The model under review builds one solid part; all positions refer to its coordinate system, in mm. A direction names the side the tool comes from. Round coordinates to 2 decimals unless told otherwise and drop trailing zeros. Order: outer loops, then holes, each group sorted by start corner. A loop starts at its lowest first (then second) coordinate and runs counter-clockwise, first axis right, second up.
1) Consider section B-B (y = -68.5). Give the boundary of the cut face in (x, z).
2) Mouldability with a two-part tool opening along Y and no side actions: class faces 1 (the face through (-125, 0.5, 27.4)), 2 (the face through (-106.171, 111.135, 1.409)), 3 (the face through (-127, 2, 23)) as pulls with the +Y half, pulls with the -Y half, needs draft (parallel to the pull), parting line crosses it, or undercut.
3) To check wall thickness, follow L1, parallel to Y at x = -126.7, z = 24; L2, parallel to X at y = -67, z = 18; L3, parallel to Z at x = 126.7, y = 0. State the ranges of each line that lie inside material, in increasing order.
4) Clearance check with flat-ended pins moving along their axes: P1, Ø2.5, axis at y = -94.29, z = 24, coming from the -X side; P2, Ø0.5, axis at x = 117, y = 110.5, coming from the +Z side; P3, Ø2.5, axis at y = 11, z = 23.5, coming from the +X side; P4, Ø8, axis at x = 91, y = 31.5, coming from the +Z side. State where each tip first meets the part, or that it passes through.
5) Consider section A-A (x = 45.5). Give the boundary of the cut face in (y, z).
6) Consider section C-C (y = 46). Give the boundary of the cut face in (x, z), then the cut area to 3 significant figures.
7) Machinability: for faces 4 (the face through (-2, 4, 0)), 5 (the face through (-127.36, 108.23, 32.19)), 6 (the face through (127, 2, 23)), which of the approach directions +Z, -Z, +X, -X, +Y, -Y give a long, thin tool a straight path to every point of the face, cutting with its end or side? Answer none if there is none.
from build123d import *

# Parameters (mm, degrees)
SKETCH1_W                                      = 255
SKETCH1_H                                      = 223
BOSS_EXTRUDE1_DEPTH                            = 2.5
SKETCH2_W                                      = 2.5
SKETCH2_H                                      = 223
SKETCH2_W_2                                    = 250
SKETCH2_H_2                                    = 2.5
BOSS_EXTRUDE2_DEPTH                            = 54
FRONT_TAPER_DEPTH                              = 178.776545135
FRONT_TAPER_DEPTH_BACK                         = 178.776545135
HOLD_IN_TAB_DEPTH                              = 3
SKETCH6_W                                      = 8.4
SKETCH6_H                                      = 227.2
MOUNTING_POCKET_DEPTH                          = 284.052115343
CSK_FOR_M3_FLAT_HEAD_MACHINE_SCREW1_AT_2_COUNT = 2
CSK_FOR_M3_FLAT_HEAD_MACHINE_SCREW1_AT_2_PITCH = 94.285714286
CSK_FOR_M3_FLAT_HEAD_MACHINE_SCREW1_AT_3_COUNT = 2
CSK_FOR_M3_FLAT_HEAD_MACHINE_SCREW1_AT_3_PITCH = 188.571428571
FILLET2_R                                      = 5
FILLET3_R                                      = 10
FILLET4_R                                      = 50
INSERT_CHAMS_SIZE                              = 1.5
INSIDE_CHAMS_SIZE                              = 2
DEBURS_SIZE                                    = 0.5


with BuildPart() as part:
    # Sketch1 → Boss-Extrude1 (new body)
    with BuildSketch(Plane.XY):
        Rectangle(SKETCH1_W, SKETCH1_H)
    extrude(amount=-BOSS_EXTRUDE1_DEPTH)

    # Sketch2 → Boss-Extrude2 (add)
    with BuildSketch(Plane.XY):
        with Locations((-126.25, 0)):
            Rectangle(SKETCH2_W, SKETCH2_H)
        with Locations((0, -110.25)):
            Rectangle(SKETCH2_W_2, SKETCH2_H_2)
        with Locations((126.25, 0)):
            Rectangle(SKETCH2_W, SKETCH2_H)
    extrude(amount=BOSS_EXTRUDE2_DEPTH)

    # Sketch5 → Front Taper (cut, two sides: drawn at the far end of the back side and taken through both)
    with BuildSketch(Plane(origin=(0, 0, 0), x_dir=(0, 0, -1), z_dir=(1, 0, 0)).offset(-FRONT_TAPER_DEPTH_BACK)):
        Polygon((-54, 31.5), (-33, 111.5), (-54, 111.5), align=None)
    extrude(amount=FRONT_TAPER_DEPTH + FRONT_TAPER_DEPTH_BACK, mode=Mode.SUBTRACT)

    # Sketch10 → Hold In Tab (add)
    with BuildSketch(Plane(origin=(0, 111.5, 0), x_dir=(1, 0, 0), z_dir=(0, 1, 0))):
        Polygon((127.5, -15), (113.5, -15), (107.5, -9), (107.5, 2.5), (127.5, 2.5), align=None)
    hold_in_tab = extrude(amount=-HOLD_IN_TAB_DEPTH)

    # Hold Tabs: Hold In Tab across plane
    add(hold_in_tab.mirror(Plane(origin=(0, 0, 0), x_dir=(0, 0, 1), z_dir=(1, 0, 0))))

    # Sketch6 → Mounting Pocket (cut, through all)
    with BuildSketch(Plane.ZY.offset(-127)):
        with Locations((24, 1.35)):
            Rectangle(SKETCH6_W, SKETCH6_H)
    mounting_pocket = extrude(amount=-MOUNTING_POCKET_DEPTH, mode=Mode.SUBTRACT)

    # Mounting Pockets: Mounting Pocket across plane
    add(mounting_pocket.mirror(Plane(origin=(0, 0, 0), x_dir=(0, 0, 1), z_dir=(1, 0, 0))), mode=Mode.SUBTRACT)

    # Sketch9 → CSK for M3 Flat Head Machine Screw1 (revolve, cut)
    with BuildSketch(Plane(origin=(125, -94.285714286, 24), x_dir=(0, 0, 1), z_dir=(0, 1, 0))):
        Polygon((0, 0), (0, 2), (1.8, 2), (1.7, 1.9), (1.7, 1.55), (3.25, 0), align=None)
    csk_for_m3_flat_head_machine_screw1 = revolve(axis=Axis((118.65, -94.285714286, 24), (1, 0, 0)), mode=Mode.SUBTRACT)

    # CSK for M3 Flat Head Machine Screw1 at 2: CSK for M3 Flat Head Machine Screw1 ×2
    with Locations(*[(0, i * CSK_FOR_M3_FLAT_HEAD_MACHINE_SCREW1_AT_2_PITCH, 0) for i in range(1, CSK_FOR_M3_FLAT_HEAD_MACHINE_SCREW1_AT_2_COUNT)]):
        add(csk_for_m3_flat_head_machine_screw1, mode=Mode.SUBTRACT)

    # CSK for M3 Flat Head Machine Screw1 at 3: CSK for M3 Flat Head Machine Screw1 ×2
    with Locations(*[(0, i * CSK_FOR_M3_FLAT_HEAD_MACHINE_SCREW1_AT_3_PITCH, 0) for i in range(1, CSK_FOR_M3_FLAT_HEAD_MACHINE_SCREW1_AT_3_COUNT)]):
        add(csk_for_m3_flat_head_machine_screw1, mode=Mode.SUBTRACT)

    # Mounting Screw Holes: CSK for M3 Flat Head Machine Screw1 across plane
    add(csk_for_m3_flat_head_machine_screw1.mirror(Plane(origin=(0, 0, 0), x_dir=(0, 0, 1), z_dir=(1, 0, 0))), mode=Mode.SUBTRACT)

    # Mounting Screw Holes copy 1 sketch → Mounting Screw Holes copy 1 (revolve, cut)
    with BuildSketch(Plane(origin=(-125, 0, 24), x_dir=(0, 0, 1), z_dir=(0, 1, 0))):
        Polygon((0, 0), (0, -2), (1.8, -2), (1.7, -1.9), (1.7, -1.55), (3.25, 0), align=None)
    revolve(axis=Axis((-118.65, 0, 24), (1, 0, 0)), mode=Mode.SUBTRACT)

    # Mounting Screw Holes copy 2 sketch → Mounting Screw Holes copy 2 (revolve, cut)
    with BuildSketch(Plane(origin=(-125, 94.285714286, 24), x_dir=(0, 0, 1), z_dir=(0, 1, 0))):
        Polygon((0, 0), (0, -2), (1.8, -2), (1.7, -1.9), (1.7, -1.55), (3.25, 0), align=None)
    revolve(axis=Axis((-118.65, 94.285714286, 24), (1, 0, 0)), mode=Mode.SUBTRACT)

    # Fillet2
    fillet2_edges = [part.edges().sort_by_distance(p)[0] for p in [
        (125, 110, 15),
        (107.5, 110, 0),
        (107.5, 110, 9),
        (113.5, 110, 15),
        (-125, 110, 15),
        (-107.5, 110, 0),
        (-107.5, 110, 9),
        (-113.5, 110, 15),
    ]]
    fillet(fillet2_edges, radius=FILLET2_R)

    # Fillet3
    fillet3_edges = [part.edges().sort_by_distance(p)[0] for p in [
        (-126.25, 111.5, 33),
        (126.25, 111.5, 33),
    ]]
    fillet(fillet3_edges, radius=FILLET3_R)

    # Fillet4
    fillet4_edges = [part.edges().sort_by_distance(p)[0] for p in [
        (126.25, 31.5, 54),
        (-126.25, 31.5, 54),
    ]]
    fillet(fillet4_edges, radius=FILLET4_R)

    # Insert Chams
    # the kernel refuses this chamfer: 1.5 mm, written as the material it takes off along each edge
    with BuildSketch(Plane(origin=(-112.035533906, 108.5, 13.535533906), x_dir=(0.01944252080601449, 0.9996219169112968, 0.01944252080601441), z_dir=(0.7071067811865461, 0, -0.707106781186549)), Plane(origin=(112.035533906, 108.5, 13.535533906), x_dir=(0.706839436070675, -0.02749587661058209, -0.7068394360706722), z_dir=(-0.7071067811865461, 0, -0.707106781186549))) as insert_chams_piece_1:
        Polygon((INSERT_CHAMS_SIZE * 0.999621916911, -INSERT_CHAMS_SIZE * 0.0274958766106), (-INSERT_CHAMS_SIZE * 0.0274958766106, -INSERT_CHAMS_SIZE * 0.999621916911), (0, 0), align=None)
    extrude(amount=4.343145751, mode=Mode.SUBTRACT)
    with BuildSketch(Plane(origin=(-107.5, 108.5, 6.928932188), x_dir=(0.027495876610582292, 0.9996219169112969, 0), z_dir=(0, 0, -1)), Plane(origin=(107.5, 108.5, 6.928932188), x_dir=(0.9996219169112969, -0.027495876610582292, 0), z_dir=(0, 0, -1))) as insert_chams_piece_2:
        Polygon((INSERT_CHAMS_SIZE * 0.999621916911, -INSERT_CHAMS_SIZE * 0.0274958766106), (-INSERT_CHAMS_SIZE * 0.0274958766106, -INSERT_CHAMS_SIZE * 0.999621916911), (0, 0), align=None)
    extrude(amount=1.928932188, mode=Mode.SUBTRACT)
    with BuildSketch(Plane(origin=(-120, 108.5, 15), x_dir=(0, 0.9996219169112968, 0.027495876610586893), z_dir=(1, 0, 0)), Plane(origin=(120, 108.5, 15), x_dir=(0, -0.027495876610582164, -0.9996219169112969), z_dir=(-1, 0, 0))) as insert_chams_piece_3:
        Polygon((INSERT_CHAMS_SIZE * 0.999621916911, -INSERT_CHAMS_SIZE * 0.0274958766106), (-INSERT_CHAMS_SIZE * 0.0274958766106, -INSERT_CHAMS_SIZE * 0.999621916911), (0, 0), align=None)
    extrude(amount=4.428932188, mode=Mode.SUBTRACT)
    with BuildSketch(Plane(origin=(-115.571067812, 108.5, 10), x_dir=(0, 0, 1), z_dir=(-1, 0, 0))) as insert_chams_piece_4:
        Polygon((5, INSERT_CHAMS_SIZE), (5 - INSERT_CHAMS_SIZE, 0), (5, 0), align=None)
    revolve(axis=Axis((-115.571067812, 108.5, 10), (0, 1, 0)), revolution_arc=45, mode=Mode.SUBTRACT)
    with BuildSketch(Plane(origin=(-112.5, 108.5, 6.928932188), x_dir=(1, 0, 0), z_dir=(0, 0, -1))) as insert_chams_piece_5:
        Polygon((5, -INSERT_CHAMS_SIZE), (5 - INSERT_CHAMS_SIZE, 0), (5, 0), align=None)
    revolve(axis=Axis((-112.5, 108.5, 6.928932188), (0, -1, 0)), revolution_arc=45, mode=Mode.SUBTRACT)
    with BuildSketch(Plane(origin=(115.571067812, 108.5, 10), x_dir=(0, 0, 1), z_dir=(1, 0, 0))) as insert_chams_piece_6:
        Polygon((5 - INSERT_CHAMS_SIZE, 0), (5, -INSERT_CHAMS_SIZE), (5, 0), align=None)
    revolve(axis=Axis((115.571067812, 108.5, 10), (0, -1, 0)), revolution_arc=45, mode=Mode.SUBTRACT)
    with BuildSketch(Plane(origin=(112.5, 108.5, 6.928932188), x_dir=(-0.7071067811865478, 0, 0.7071067811865472), z_dir=(0.7071067811865472, 0, 0.7071067811865478))) as insert_chams_piece_7:
        Polygon((5 - INSERT_CHAMS_SIZE, 0), (5, -INSERT_CHAMS_SIZE), (5, 0), align=None)
    revolve(axis=Axis((112.5, 108.5, 6.928932188), (0, -1, 0)), revolution_arc=45, mode=Mode.SUBTRACT)
    with BuildSketch(Plane(origin=(-120, 108.5, 20), x_dir=(-0.7166461305573681, 0, 0.6974369674437623), z_dir=(0.6974369674437623, 0, 0.7166461305573681))) as insert_chams_piece_8_section:
        Polygon((5, -INSERT_CHAMS_SIZE), (5 + INSERT_CHAMS_SIZE, 0), (5, 0), align=None)
    insert_chams_piece_8 = revolve(axis=Axis((-120, 108.5, 20), (0, -1, 0)), revolution_arc=134.221731534, mode=Mode.PRIVATE)
    insert_chams_piece_8 = split(insert_chams_piece_8, bisect_by=Plane(origin=(-125, 109.058393583, 16.326998509), z_dir=(1, 0, 0)), keep=Keep.TOP, mode=Mode.PRIVATE)
    add(insert_chams_piece_8, mode=Mode.SUBTRACT)
    with BuildSketch(Plane(origin=(-102.5, 108.5, 5), x_dir=(0.6974369674437586, 0, -0.7166461305573718), z_dir=(0.7166461305573718, 0, 0.6974369674437586))) as insert_chams_piece_9_section:
        Polygon((5, INSERT_CHAMS_SIZE), (5 + INSERT_CHAMS_SIZE, 0), (5, 0), align=None)
    insert_chams_piece_9 = revolve(axis=Axis((-102.5, 108.5, 5), (0, 1, 0)), revolution_arc=134.221731534, mode=Mode.PRIVATE)
    insert_chams_piece_9 = split(insert_chams_piece_9, bisect_by=Plane(origin=(-106.173001491, 109.058393583, 0), z_dir=(0, 0, 1)), keep=Keep.TOP, mode=Mode.PRIVATE)
    add(insert_chams_piece_9, mode=Mode.SUBTRACT)
    with BuildSketch(Plane(origin=(102.5, 108.5, 5), x_dir=(-0.6974369674437586, 0, -0.7166461305573718), z_dir=(-0.7166461305573718, 0, 0.6974369674437586))) as insert_chams_piece_10_section:
        Polygon((5 + INSERT_CHAMS_SIZE, 0), (5, -INSERT_CHAMS_SIZE), (5, 0), align=None)
    insert_chams_piece_10 = revolve(axis=Axis((102.5, 108.5, 5), (0, -1, 0)), revolution_arc=134.221731534, mode=Mode.PRIVATE)
    insert_chams_piece_10 = split(insert_chams_piece_10, bisect_by=Plane(origin=(106.173001491, 109.058393583, 0), z_dir=(0, 0, 1)), keep=Keep.TOP, mode=Mode.PRIVATE)
    add(insert_chams_piece_10, mode=Mode.SUBTRACT)
    with BuildSketch(Plane(origin=(120, 108.5, 20), x_dir=(0.716646130557371, 0, 0.6974369674437595), z_dir=(-0.6974369674437595, 0, 0.716646130557371))) as insert_chams_piece_11_section:
        Polygon((5, INSERT_CHAMS_SIZE), (5 + INSERT_CHAMS_SIZE, 0), (5, 0), align=None)
    insert_chams_piece_11 = revolve(axis=Axis((120, 108.5, 20), (0, 1, 0)), revolution_arc=134.221731534, mode=Mode.PRIVATE)
    insert_chams_piece_11 = split(insert_chams_piece_11, bisect_by=Plane(origin=(125, 109.058393583, 16.326998509), z_dir=(-1, 0, 0)), keep=Keep.TOP, mode=Mode.PRIVATE)
    add(insert_chams_piece_11, mode=Mode.SUBTRACT)

    # Inside Chams
    inside_chams_edges = [part.edges().sort_by_distance(p)[0] for p in [
        (-125, -109, 27),
        (125, -109, 27),
        (0, -109, 0),
        (-125, 108.5, 7.923344034),
        (-115.826655966, 108.5, 0),
        (125, 108.5, 7.923344034),
        (125, -0.25, 0),
        (115.826655966, 108.5, 0),
        (-125, -0.25, 0),
    ]]
    chamfer(inside_chams_edges, length=INSIDE_CHAMS_SIZE)

    # Deburs
    deburs_edges = [part.edges().sort_by_distance(p)[0] for p in [
        (-127.5, 0, -2.5),
        (0, -111.5, -2.5),
        (0, -111.5, 54),
        (-110.5, 111.5, 12),
        (-117.785533906, 111.5, 15),
        (-107.5, 111.5, 5.964466094),
        (0, 111.5, 0),
        (107.5, 111.5, 5.964466094),
        (110.5, 111.5, 12),
        (117.785533906, 111.5, 15),
        (113.65765065, 111.5, 14.619397663),
        (107.880602337, 111.5, 8.84234935),
        (-113.65765065, 111.5, 14.619397663),
        (-107.880602337, 111.5, 8.84234935),
        (-123.535533906, 111.5, 16.464466094),
        (-106.035533906, 111.5, 1.464466094),
        (106.035533906, 111.5, 1.464466094),
        (123.535533906, 111.5, 16.464466094),
        (125, 111.5, 22.64310388),
        (-125, 111.5, 22.64310388),
        (-125, 109.418011519, 31.393997341),
        (-127.5, 108.431990614, 32.493669596),
        (127.5, 108.431990614, 32.493669596),
        (125, 109.418011519, 31.393997341),
        (-125, 70.890351082, 43.660032841),
        (-127.5, 70.890351082, 43.660032841),
        (-125, -40.97659277, 54),
        (-125, 31.446915496, 53.588695352),
        (-127.5, -43.22659277, 54),
        (127.5, -43.22659277, 54),
        (125, -40.97659277, 54),
        (-127.5, 31.446915496, 53.588695352),
        (127.5, 70.890351082, 43.660032841),
        (125, 70.890351082, 43.660032841),
        (127.5, 31.446915496, 53.588695352),
        (125, 31.446915496, 53.588695352),
        (0, -109, 54),
        (-124, -108, 54),
        (124, -108, 54),
        (127.5, 0, -2.5),
        (127.5, -111.5, 8.65),
        (-127.5, -111.5, 8.65),
        (-127.5, 111.5, 8.65),
        (127.5, 111.5, 8.65),
        (0, 111.5, -2.5),
    ]]
    chamfer(deburs_edges, length=DEBURS_SIZE)


solid = part.part
Answer below:
1. outline: (-127.5, -2) - (-127, -2.5) - (127, -2.5) - (127.5, -2) - (127.5, 19.8) - (127, 19.8) - (127, 28.2) - (127.5, 28.2) - (127.5, 53.5) - (127, 54) - (125.5, 54) - (125, 53.5) - (125, 2) - (123, 0) - (-123, 0) - (-125, 2) - (-125, 53.5) - (-125.5, 54) - (-127, 54) - (-127.5, 53.5) - (-127.5, 28.2) - (-127, 28.2) - (-127, 19.8) - (-127.5, 19.8) - close
2. face 1: undercut
2. face 2: pulls with the +Y half
2. face 3: needs draft
3. L1: y = -111.5 to -95.99, -92.59 to -1.7, 1.7 to 92.59, 95.99 to 111.5
3. L2: x = -127.5 to -125, 125 to 127.5
3. L3: z = -2.5 to 22.3, 25.7 to 54
4. P1: passes through
4. P2: stops at z = 15
4. P3: stops at x = 127
4. P4: stops at z = 0
5. outline: (-111.5, -2) - (-111, -2.5) - (111, -2.5) - (111.5, -2) - (111.5, -0.5) - (111, 0) - (-107, 0) - (-109, 2) - (-109, 53.5) - (-109.5, 54) - (-111, 54) - (-111.5, 53.5) - close
6. outline: (-127.5, -2) - (-127, -2.5) - (127, -2.5) - (127.5, -2) - (127.5, 19.8) - (127, 19.8) - (127, 28.2) - (127.5, 28.2) - (127.5, 49.68) - (127, 50.19) - (125.5, 50.19) - (125, 49.68) - (125, 2) - (123, 0) - (-123, 0) - (-125, 2) - (-125, 49.68) - (-125.5, 50.19) - (-127, 50.19) - (-127.5, 49.68) - (-127.5, 28.2) - (-127, 28.2) - (-127, 19.8) - (-127.5, 19.8) - close
6. area: 883 mm2
7. face 4: +Z
7. face 5: +Z, -X, +Y
7. face 6: +X, +Y, -Y
